Here's how the part is built. I have some questions about the finished solid (model axes, mm). Round coordinates to 2 decimals unless told otherwise and drop trailing zeros. Loops run counter-clockwise (first coordinate to the right, second up) from the corner with the lowest first, then second, coordinate; pieces in that order, holes last. Notation, with made-up numbers: M 50,43.25 L 82,43.25 A18 ccw 82,54.25 Z; hole C 63,-18 d1. An arc over 180 degrees is marked long. Use a Markdown table: item, result.
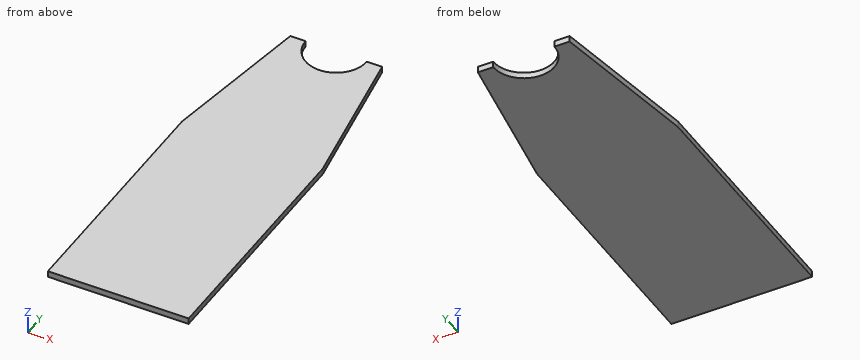
Autodesk Inventor part; units mm, degrees
ref_plane "YZ Plane" through (0, 0, 0) normal (1, 0, 0) x (0, 1, 0)
ref_plane "XZ Plane" through (0, 0, 0) normal (0, 1, 0) x (-1, 0, 0)
ref_plane "XY Plane" through (0, 0, 0) normal (0, 0, 1) x (1, 0, 0)
sketch "Sketch1" plane through (0, 0, 0) normal (0, 0, 1) x (1, 0, 0)
  line L0 (115, 200) -> (115, -200)
  line L1 (115, -200) -> (-115, -200)
  line L2 (-115, -200) -> (-115, 200)
  arc A0 (-50, 450) -> (50, 450) centre (0, 450) ccw
  line L3 (-115, 200) -> (-75, 450)
  line L4 (75, 450) -> (115, 200)
  line L5 (-75, 450) -> (-50, 450)
  line L6 (50, 450) -> (75, 450)
  point P0 (0, 0)
  dimension "d1" = 400
  dimension "d2" = 115
  dimension "d3" = 200
  dimension "d6" = 100
  dimension "d9" = 150
  dimension "d10" = 25
  dimension "d11" = 25
  dimension "d14" = 450
  dimension "d15" = 230
  dimension "d16" = 170.91
  dimension "d17" = 170.91
  dimension "d18" = 450
  dimension "d19" = 450
  dimension "d20" = 115
extrude "Extrusion1" add sketch "Sketch1" along normal blind 10
properties part number "Suporte" material "Lead"
1. For pin 1 Ø4 at (y, z) = (244.5, 4) entering from -X, with a flat end and sliding along its axis, tell me the tip position at first contact or that it passes through.
Answer sheet:
| item | result |
|---|---|
| pin 1 | x = -108.2 |
2. Imagine slicing it at B-B, the plane x = 0. Write out the boundary of the cut face in (y, z), then the cut area to 3 significant figures.
Answer sheet:
| item | result |
|---|---|
| outline | M -200,0 L 400,0 L 400,10 L -200,10 Z |
| area | 6,000 mm2 |
3. Imagine slicing it at C-C, the plane y = 289.5. Write out the boundary of the cut face in (x, z), then the cut area to 3 significant figures.
Answer sheet:
| item | result |
|---|---|
| outline | M -100.68,0 L 100.68,0 L 100.68,10 L -100.68,10 Z |
| area | 2,010 mm2 |
4. I need wall thicknesses on probe 1 along Y at (x, z) = (-1, 9.5); probe 2 along Y at (x, z) = (-20.5, 6); probe 3 along X at (y, z) = (266, 9.5). Which ranges of each line are inside material? Lowest first, please. Write a range as from..to.
Answer sheet:
| item | result |
|---|---|
| probe 1 | -200..400.01 |
| probe 2 | -200..404.4 |
| probe 3 | -104.44..104.44 |
5. Imagine slicing it at A-A, the plane z = 2.75. Write out the boundary of the cut face in (x, y), then the cut area to 3 significant figures.
Answer sheet:
| item | result |
|---|---|
| outline | M -115,-200 L 115,-200 L 115,200 L 75,450 L 50,450 A50 cw -50,450 L -75,450 L -115,200 Z |
| area | 136,000 mm2 |
